Autodesk Inventor part; units mm, degrees
ref_plane "YZ Plane" through (0, 0, 0) normal (1, 0, 0) x (0, 1, 0)
ref_plane "XZ Plane" through (0, 0, 0) normal (0, 1, 0) x (-1, 0, 0)
ref_plane "XY Plane" through (0, 0, 0) normal (0, 0, 1) x (1, 0, 0)
sketch "Sketch1" plane through (0, 0, 0) normal (0, 1, 0) x (-1, 0, 0)
  line L0 (-10, -10) -> (10, -10)
  line L1 (10, -10) -> (10, 10)
  line L2 (10, 10) -> (-10, 10)
  line L3 (-10, 10) -> (-10, -10)
  line L4 (-10, -10) -> (10, 10) construction
  line L5 (10, -10) -> (-10, 10) construction
  point P0 (0, 0)
  dimension "d0" = 20
  dimension "d1" = 20
extrude "Extrusion1" add sketch "Sketch1" along normal blind 1
sketch "Sketch2" plane through (0, 1, 0) normal (0, 1, 0) x (1, 0, 0)
  line L0 (-10, -10) -> (10, -10)
  line L1 (10, 10) -> (-10, 10)
  line L2 (-10, -10) -> (-9, -10)
  line L3 (-9, -10) -> (-9, 10)
  line L4 (-9, 10) -> (-10, 10)
  line L5 (-10, 10) -> (-10, -10)
  point P0 (0, 0)
  dimension "d4" = 1
extrude "Extrusion2" add sketch "Sketch2" along normal blind 19
sketch "Sketch3" plane through (-10, 0, -10) normal (-1, 0, 0) x (0, 0, 1)
  circle A0 centre (10, 12) radius 2
  point P0 (10, 0)
  dimension "d7" = 4
extrude "Extrusion3" cut sketch "Sketch3" against normal blind 10
sketch "Sketch4" plane through (0, 0, 0) normal (0, -1, 0) x (1, 0, 0)
  circle A0 centre (2, 0) radius 2
  point P0 (0, 0)
extrude "Extrusion4" cut sketch "Sketch4" against normal blind 10
properties part number "trail 11"
Geometry: final body of the model. Coordinates: model frame, mm. A direction names the side the tool comes from. Give positions to 0.01 mm unless a question says otherwise; leave off trailing zeros. Write each loop counter-clockwise with the first axis right and the second up, starting at its lowest first coordinate (ties: lowest second). Pieces come first, ordered by that corner, then holes.
(1) Ray query, line 1 (Z direction, x = 2, y = 0.45); line 2 (Y direction, x = -9.7, z = 0); line 3 (X direction, y = 9, z = -1.5). Return the intervals inside material, ascending.
(2) Cut plane A-A, the plane y = 12. Return loops of the section in (x, z).
(3) Mould query, pull axis X, two halves, no side actions, for faces 1 (the flat face through (-9, 8, 0)), 2 (the flat face through (-4.5, 0.3, 10)), 3 (the cylindrical face through (1.566, 0.493, -1.952)). Classes: released by +X, released by -X, zero draft, split by the parting line, or undercut.
(4) Access query for faces 4 (the flat face through (10, 0.5, 0.1)), 5 (the flat face through (-1, 1, 0)). Directions: +Z, -Z, +X, -X, +Y, -Y. A direction counts if a zero-diameter tool reaches every point of the face in a straight line with its end or side. Return the directions, or none.
(5) Cut plane C-C, the plane z = 0. Return loops of the section in (x, y), then the cut area to 3 significant figures.
(6) Cut plane D-D, the plane z = -4. Return loops of the section in (x, y), then the cut area to 3 significant figures.
(7) First-contact query: P1, Ø5, axis at y = 12, z = 0, coming from the +X side; P2, Ø5, axis at x = 2, z = 0, coming from the +Y side. Flat tips, straight axial feed; report the tip coordinate or a pass-through.
(8) Cut plane B-B, the plane x = 2. Return loops of the section in (y, z), then the cut area to 3 significant figures.
Values follow:
1. line 1: z = -10 to -2, 2 to 10
1. line 2: y = 0 to 10, 14 to 20
1. line 3: x = -10 to -9
2. outline: (-10, -10) - (-9, -10) - (-9, -2) - (-10, -2) - close; (-10, 2) - (-9, 2) - (-9, 10) - (-10, 10) - close
3. face 1: released by +X
3. face 2: zero draft
3. face 3: undercut
4. face 4: +Z, -Z, +X, +Y, -Y
4. face 5: +Z, -Z, +X, +Y
5. outline: (-10, 0) - (0, 0) - (0, 1) - (-9, 1) - (-9, 10) - (-10, 10) - close; (-10, 14) - (-9, 14) - (-9, 20) - (-10, 20) - close; (4, 0) - (10, 0) - (10, 1) - (4, 1) - close
5. area: 31.0 mm2
6. outline: (-10, 0) - (10, 0) - (10, 1) - (-9, 1) - (-9, 20) - (-10, 20) - close
6. area: 39.0 mm2
7. P1: stops at x = -9
7. P2: stops at y = 1
8. outline: (0, -10) - (1, -10) - (1, -2) - (0, -2) - close; (0, 2) - (1, 2) - (1, 10) - (0, 10) - close
8. area: 16.0 mm2
